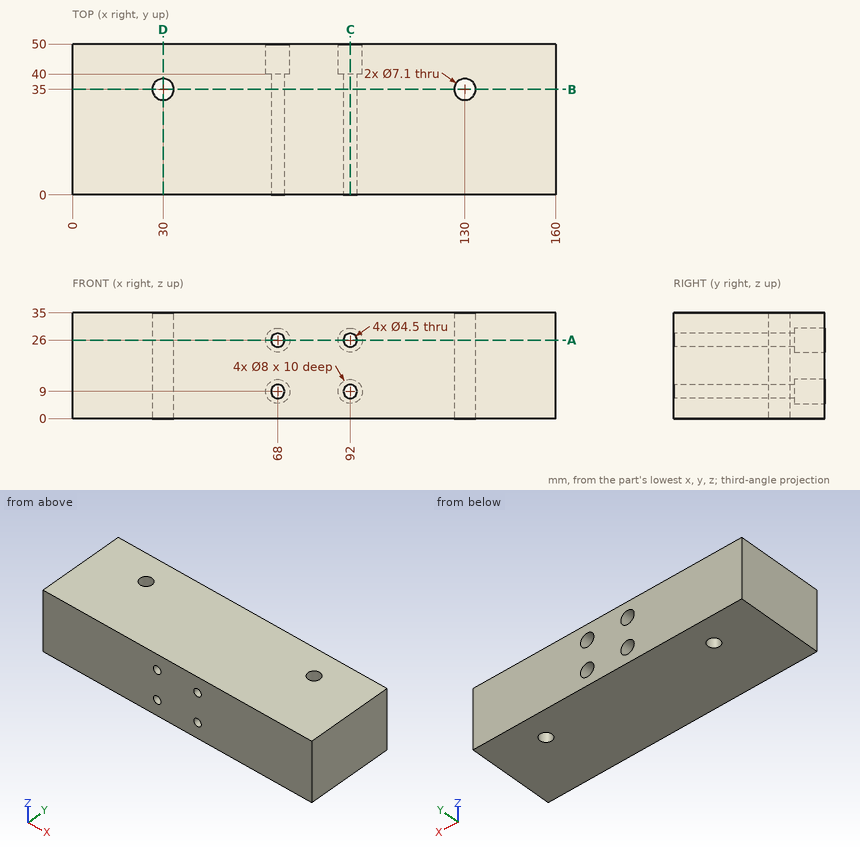
Print and shaded views of the part. All mm, measured from the part's lowest x, y and z. Coordinates: 2 decimals unless noted, no trailing zeros. Write each loop counter-clockwise with the first axis right and the second up, starting at its lowest first coordinate (ties: lowest second). Pieces come first, ordered by that corner, then holes.
(1) Cut at B-B, the plane y = 35. List the corners of the cut face in (x, z).
(2) Flat gauge pins, fed straight in: pin 1 (4 mm diameter, centred on x = 92, z = 9, fed in from -Y); pin 2 (6.5 mm diameter, centred on x = 68, z = 25.5, fed in from +Y). Where does each tip first touch, or does it go through?
(3) Cut at D-D, the plane x = 30. List the corners of the cut face in (y, z).
(4) Cut at C-C, the plane x = 92. List the corners of the cut face in (y, z), and give its area (3 significant figures).
(5) Drill centre lines: probe 1 along X at (y, z) = (42.75, 9); probe 2 along Z at (x, y) = (92, 9.5); probe 3 along X at (y, z) = (11.5, 24). Where is each one in solid material? Low to high.
(6) Cut at A-A, the plane z = 26. List the corners of the cut face in (x, y).
Geometry says:
1. outline: (0, 0) - (26.45, 0) - (26.45, 35) - (0, 35) - close; (33.55, 0) - (126.45, 0) - (126.45, 35) - (33.55, 35) - close; (133.55, 0) - (160, 0) - (160, 35) - (133.55, 35) - close; hole circle Ø4.5 at (68, 9); hole circle Ø4.5 at (68, 26); hole circle Ø4.5 at (92, 9); hole circle Ø4.5 at (92, 26)
2. pin 1: passes through
2. pin 2: stops at y = 40
3. outline: (0, 0) - (31.45, 0) - (31.45, 35) - (0, 35) - close; (38.55, 0) - (50, 0) - (50, 35) - (38.55, 35) - close
4. outline: (0, 0) - (50, 0) - (50, 5) - (40, 5) - (40, 6.75) - (0, 6.75) - close; (0, 11.25) - (40, 11.25) - (40, 13) - (50, 13) - (50, 22) - (40, 22) - (40, 23.75) - (0, 23.75) - close; (0, 28.25) - (40, 28.25) - (40, 30) - (50, 30) - (50, 35) - (0, 35) - close
4. area: 1,230 mm2
5. probe 1: x = 0 to 64, 72 to 88, 96 to 160
5. probe 2: z = 0 to 6.75, 11.25 to 23.75, 28.25 to 35
5. probe 3: x = 0 to 66.97, 69.03 to 90.97, 93.03 to 160
6. outline: (0, 0) - (65.75, 0) - (65.75, 40) - (64, 40) - (64, 50) - (0, 50) - close; (70.25, 0) - (89.75, 0) - (89.75, 40) - (88, 40) - (88, 50) - (72, 50) - (72, 40) - (70.25, 40) - close; (94.25, 0) - (160, 0) - (160, 50) - (96, 50) - (96, 40) - (94.25, 40) - close; hole circle Ø7.1 at (30, 35); hole circle Ø7.1 at (130, 35)
